from build123d import *

# Parameters (mm, degrees)
F1_DEPTH  = 1.6
F3_DEPTH  = 8.24
F5_DEPTH  = 12.5
F7_DEPTH  = 7
F9_DEPTH  = 2
F10_R     = 1.5
F11_DEPTH = 18.4
F12_R     = 0.5
F13_DEPTH = 7
F14_R     = 0.5
F15_DEPTH = 7
F17_DEPTH = 1.6
F20_R     = 5
F22_DEPTH = 9.4
F24_DEPTH = 7.5
F25_R     = 4.6
F26_DEPTH = 2.5
F27_R     = 0.5
F28_DEPTH = 7


with BuildPart() as f1:
    # F0 (on Top) → F1 (new body)
    with BuildSketch(Plane.XY):
        Polygon((-25, 20.5), (-40, 20.5), (-40, -20.5), (-25, -20.5), (0, -20.5), (25, -20.5), (40, -20.5), (40, 20.5), (25, 20.5), (0, 20.5), align=None)
        Polygon((-25, 30), (-25, 20.5), (0, 20.5), (25, 20.5), (25, 30), align=None)
        Polygon((0, -20.5), (-25, -20.5), (-25, -30), (25, -30), (25, -20.5), align=None)
    extrude(amount=F1_DEPTH)

    # F2 (on face) → F3 (join)
    with BuildSketch(Plane.XY.offset(1.6)):
        Polygon((40, -12.75), (40, 0), (40, 12.75), (33.5, 12.75), (33.5, -12.75), align=None)
        Polygon((40, 12.75), (40, 0), (40, -12.75), (45.5, -12.75), (45.5, 12.75), align=None)
    extrude(amount=F3_DEPTH)

    # F4 (on face) → F5 (join)
    with BuildSketch(Plane.XY.offset(1.6)):
        Polygon((-40, -15.5), (-40, 0), (-40, 15.5), (-43, 15.5), (-43, -15.5), align=None)
        Polygon((-40, 15.5), (-40, 0), (-40, -15.5), (-31, -15.5), (-31, 15.5), align=None)
    extrude(amount=F5_DEPTH)

    # F6 (on face) → F7 (join)
    with BuildSketch(Plane(origin=(-43, 0, 0), x_dir=(0, -1, 0), z_dir=(-1, 0, 0))):
        Polygon((0, 11.6), (0, 3.6), (5, 3.6), (8, 11.6), align=None)
        Polygon((-5, 3.6), (0, 3.6), (0, 11.6), (-8, 11.6), align=None)
        Polygon((-14, 10.4480762114), (-15.5, 7.85), (-14, 5.2519237886), (-11, 5.2519237886), (-9.5, 7.85), (-11, 10.4480762114), align=None)
        Polygon((15.0980762114, 9.35), (12.5, 10.85), (9.9019237886, 9.35), (9.9019237886, 6.35), (12.5, 4.85), (15.0980762114, 6.35), (15.0980762114, 7.85), align=None)
    extrude(amount=F7_DEPTH)

    # F8 (on face) → F9 (cut)
    with BuildSketch(Plane.XY.offset(1.6)):
        with BuildLine():
            ThreePointArc((37.7, 16.5), (37.2606601718, 17.5606601718), (36.2, 18))
            Line((36.2, 18), (36.2, 16.5))
            Line((36.2, 16.5), (36.2, 15))
            ThreePointArc((36.2, 15), (37.2606601718, 15.4393398282), (37.7, 16.5))
        make_face()
        with BuildLine():
            ThreePointArc((-23.3, -16.5), (-25.8606601718, -15.4393398282), (-24.8, -18))
            ThreePointArc((-24.8, -18), (-23.7393398282, -17.5606601718), (-23.3, -16.5))
        make_face()
        with BuildLine():
            ThreePointArc((37.7, -16.5), (37.2606601718, -15.4393398282), (36.2, -15))
            Line((36.2, -15), (36.2, -16.5))
            Line((36.2, -16.5), (36.2, -18))
            ThreePointArc((36.2, -18), (37.2606601718, -17.5606601718), (37.7, -16.5))
        make_face()
        with BuildLine():
            Line((36.2, -16.5), (36.2, -15))
            ThreePointArc((36.2, -15), (34.7, -16.5), (36.2, -18))
            Line((36.2, -18), (36.2, -16.5))
        make_face()
        with BuildLine():
            Line((36.2, 16.5), (36.2, 18))
            ThreePointArc((36.2, 18), (34.7, 16.5), (36.2, 15))
            Line((36.2, 15), (36.2, 16.5))
        make_face()
        with BuildLine():
            ThreePointArc((-24.8, 18), (-25.8606601718, 15.4393398282), (-23.3, 16.5))
            ThreePointArc((-23.3, 16.5), (-23.7393398282, 17.5606601718), (-24.8, 18))
        make_face()
    extrude(amount=-F9_DEPTH, mode=Mode.SUBTRACT)

    # F10 (on face) → F11 (join)
    with BuildSketch(Plane.XY.offset(1.6)):
        with BuildLine():
            ThreePointArc((-10.7, 21.2), (-9.6393398282, 21.6393398282), (-9.2, 22.7))
            Line((-9.2, 22.7), (-10.7, 22.7))
            Line((-10.7, 22.7), (-10.7, 21.2))
        make_face()
        with BuildLine():
            ThreePointArc((-4.5, 24.2), (-5.5606601718, 23.7606601718), (-6, 22.7))
            Line((-6, 22.7), (-4.5, 22.7))
            Line((-4.5, 22.7), (-4.5, 24.2))
        make_face()
        with BuildLine():
            Line((-4.5, 22.7), (-6, 22.7))
            ThreePointArc((-6, 22.7), (-4.5, 21.2), (-3, 22.7))
            ThreePointArc((-3, 22.7), (-3.4393398282, 23.7606601718), (-4.5, 24.2))
            Line((-4.5, 24.2), (-4.5, 22.7))
        make_face()
        with BuildLine():
            Line((-10.7, 22.7), (-9.2, 22.7))
            ThreePointArc((-9.2, 22.7), (-10.7, 24.2), (-12.2, 22.7))
            Line((-12.2, 22.7), (-10.7, 22.7))
        make_face()
        with Locations((-16.9, 22.7)):
            Circle(F10_R)
        with BuildLine():
            Line((-10.7, 21.2), (-10.7, 22.7))
            Line((-10.7, 22.7), (-12.2, 22.7))
            ThreePointArc((-12.2, 22.7), (-11.7606601718, 21.6393398282), (-10.7, 21.2))
        make_face()
    extrude(amount=F11_DEPTH)

    # F12 (on face) → F13 (join)
    with BuildSketch(Plane.XY.offset(20)):
        with Locations((-10.7, 22.7)):
            Circle(F12_R)
    extrude(amount=F13_DEPTH)

    # F14 (on face) → F15 (join)
    with BuildSketch(Plane.XY.offset(20)):
        with Locations((-4.5, 22.7)):
            Circle(F14_R)
    extrude(amount=F15_DEPTH)

    # F20
    f20_edges = [f1.edges().sort_by_distance(p)[0] for p in [
        (-25, 20.5, 0.8),
        (25, 20.5, 0.8),
        (25, -20.5, 0.8),
        (-25, -20.5, 0.8),
    ]]
    fillet(f20_edges, radius=F20_R)

    # F21 (on face) → F22 (join)
    with BuildSketch(Plane.XY.offset(1.6)):
        Polygon((21.5, 28.5), (18.5, 28.5), (15.5, 28.5), (15.5, 22.5), (21.5, 22.5), align=None)
    extrude(amount=F22_DEPTH)

    # F23 (on face) → F24 (join)
    with BuildSketch(Plane(origin=(0, 28.5, 0), x_dir=(-1, 0, 0), z_dir=(0, 1, 0))):
        with BuildLine():
            ThreePointArc((-18.5, 11), (-20.6213203436, 5.8786796564), (-15.5, 8))
            ThreePointArc((-15.5, 8), (-16.3786796564, 10.1213203436), (-18.5, 11))
        make_face()
    extrude(amount=F24_DEPTH)

    # F25 (on face) → F26 (join, symmetric)
    with BuildSketch(Plane(origin=(0, 36, 0), x_dir=(-1, 0, 0), z_dir=(0, 1, 0))):
        with Locations((-18.5, 8)):
            Circle(F25_R)
    extrude(amount=F26_DEPTH, both=True)

    # F27 (on face) → F28 (join)
    with BuildSketch(Plane.XY.offset(20)):
        with Locations((-16.9, 22.7)):
            Circle(F27_R)
    extrude(amount=F28_DEPTH)


with BuildPart() as f17:
    # F16 (on face) → F17 (new body)
    with BuildSketch(Plane.XY.offset(1.6)):
        Polygon((-57.5, 30), (-57.5, 20.5), (-32.5, 20.5), (-7.5, 20.5), (-7.5, 30), align=None)
    extrude(amount=-F17_DEPTH)


with BuildPart() as f17b:
    # F16 (on face) → F17, piece 2 (new body)
    with BuildSketch(Plane.XY.offset(1.6)):
        Polygon((-7.5, -20.5), (-32.5, -20.5), (-57.5, -20.5), (-57.5, -31.8096540868), (-7.5, -31.8096540868), align=None)
    extrude(amount=-F17_DEPTH)


solid = f1.part
Check sheet for the modelled part. Datum: model origin and axes. Units: mm. A direction names the side the tool comes from. Round coordinates to 2 decimals unless told otherwise and drop trailing zeros. Loops run counter-clockwise (first coordinate to the right, second up) from the corner with the lowest first, then second, coordinate; pieces in that order, holes last.
1. Mould release check, pull along Y, two halves, no side actions. Record for faces 4 (the flat face through (19, 38.5, 8)), 5 (the flat face through (15, 33.5, 8)), 6 (the flat face through (-46, 13, 5.252)), 7 (the flat face through (21, 28.5, 10)): released by +Y, released by -Y, zero draft, split by the parting line, or undercut.
2. Gauge pin test, flat ends, axial feed: pin 1 Ø8 at (x, z) = (-13, 21) entering from -Y; pin 2 Ø10 at (x, y) = (-26, -23) entering from +Z; pin 3 Ø4 at (y, z) = (27.5, 12) entering from -X; pin 4 Ø8 at (y, z) = (-12.5, 2.5) entering from -X. Record the tip position at first contact, or that the pin passes through.
3. Scan lines: probe 1 along Y at (x, z) = (-24.8, 0.7); probe 2 along X at (y, z) = (16.5, 1.15); probe 3 along X at (y, z) = (-9.5, 6). Record each from-to range of solid material in increasing order.
4. Set-up check for faces 1 (the flat face through (-46.45, 10.26, 6.53)), 2 (the flat face through (-46.5, -11.2, 10.1)), 3 (the cylindrical face through (22.15, 36.03, 5.2)): record each of +Z, -Z, +X, -X, +Y, -Y from which the full face is reachable in a straight line by a thin tool's end or side.
5. Sectioned sample at A-A on z = 17.75. Record the boundary of the cut face in (x, y), and give its area (3 significant figures).
6. Sectioned sample at B-B on z = 24. Record the boundary of the cut face in (x, y), and give its area (3 significant figures).
Recorded:
1. face 4: released by +Y
1. face 5: undercut
1. face 6: zero draft
1. face 7: undercut
2. pin 1: stops at y = 21.2
2. pin 2: stops at z = 1.6
2. pin 3: stops at x = 15.5
2. pin 4: stops at x = -50
3. probe 1: y = -30 to -18, -15 to 15, 18 to 30
3. probe 2: x = -40 to -26.3, -23.3 to 34.7, 37.7 to 40
3. probe 3: x = -43 to -31, 33.5 to 45.5
4. face 1: -Z, -X
4. face 2: +Z, -X
4. face 3: +Y
5. outline: circle Ø3 at (-16.9, 22.7); circle Ø3 at (-10.7, 22.7); circle Ø3 at (-4.5, 22.7)
5. area: 21.2 mm2
6. outline: circle Ø1 at (-16.9, 22.7); circle Ø1 at (-10.7, 22.7); circle Ø1 at (-4.5, 22.7)
6. area: 2.36 mm2
